```python
from build123d import *

# Parameters (mm, degrees)
EXTRUDE_1_DEPTH     = 3
SKETCH_2_R          = 2.5
CUT_EXTRUDE_1_DEPTH = 3


with BuildPart() as part:
    # 草图1 → 凸台-拉伸1 (new body)
    with BuildSketch(Plane(origin=(0, 0, 0), x_dir=(1, 0, 0), z_dir=(0, 1, 0))):
        with BuildLine():
            ThreePointArc((6.796232726, -80.103971167), (3.309364716, -83.445468492), (6.479618851, -87.088728243))
            ThreePointArc((6.479618851, -87.088728243), (23.201931583, -85.196198653), (37.766812343, -76.765204654))
            ThreePointArc((37.766812343, -76.765204654), (38.146329718, -71.950662158), (33.355557274, -71.3404554))
            ThreePointArc((33.355557274, -71.3404554), (20.773998873, -77.837935766), (6.796232726, -80.103971167))
        make_face()
    extrude(amount=EXTRUDE_1_DEPTH)

    # 草图2 → 切除-拉伸1 (cut)
    with BuildSketch(Plane(origin=(0, 0, 0), x_dir=(1, 0, 0), z_dir=(0, 1, 0))):
        with Locations(Location((6.805774449, -83.603958161, 0), (0, 0, 270))):
            Circle(SKETCH_2_R)
        with Locations(Location((35.430824241, -74.158835612, 0), (0, 0, 270))):
            Circle(SKETCH_2_R)
    extrude(amount=CUT_EXTRUDE_1_DEPTH, mode=Mode.SUBTRACT)


solid = part.part
```
The model under review builds one solid part; all positions refer to its coordinate system, in mm. Round coordinates to 2 decimals unless told otherwise and drop trailing zeros. Loops run counter-clockwise (first coordinate to the right, second up) from the corner with the lowest first, then second, coordinate; pieces in that order, holes last. Notation, with made-up numbers: M 50,-18.75 L 104,-18.75 A16 cw 104,1.25 Z; hole C 23,-25 d5. An arc over 180 degrees is marked long. Write item = value, one per line.
Item 1: Take a section at C-C on y = 2.65. Write out the cut boundary in (x, z).
Return value:
outline = M 6.48,87.09 A3.5 ccw 6.8,80.1 A45 cw 33.36,71.34 A3.5 ccw 37.77,76.77 A41.13 ccw Z; hole C 6.81,83.6 d5; hole C 35.43,74.16 d5
Item 2: Take a section at B-B on x = 5. Write out the cut boundary in (y, z).
Return value:
outline = M 0,80.61 L 3,80.61 L 3,81.88 L 0,81.88 Z; M 0,85.33 L 3,85.33 L 3,86.6 L 0,86.6 Z
Item 3: For line 1 (X direction, y = 1.2, z = 83.5); line 2 (X direction, y = 0.95, z = 76.25); line 3 (Z direction, x = 36.5, y = 1.55), list the stretches that pass through material, from the lowest coordinate up. Write a range as [from, to].
Return value:
line_1 = [3.31, 4.31], [9.3, 27.51]
line_2 = [24.89, 34.06], [36.8, 38.24]
line_3 = [70.83, 71.9], [76.42, 77.86]
Item 4: Take a section at D-D on x = 20. Write out the cut boundary in (y, z).
Return value:
outline = M 0,78.09 L 3,78.09 L 3,86.11 L 0,86.11 Z
Item 5: The part is to be moulded in two halves that separate along Z. For faces 1 (the flat face through (21, 3, 81)), 2 (the cylindrical face through (7.557, 1.479, 85.989)), 3 (the cylindrical face through (22.98, 1.48, 85.27)), say which applies: released by +Z, released by -Z, zero draft, split by the parting line, or undercut.
Return value:
face_1 = zero draft
face_2 = undercut
face_3 = released by +Z
Item 6: Insertion check: P1, Ø4, axis at x = 35.43, z = 74.16, coming from the +Y side; P2, Ø1.5, axis at x = 27, y = 2.5, coming from the +Z side. Each pin has a flat end and moves straight along its axis. Give the tip position at first contact, or say it passes through.
Return value:
P1 = through
P2 = 84.05
Item 7: Take a section at A-A on z = 75. Write out the cut boundary in (x, y), then the cut area to 3 significant figures.
Return value:
outline = M 27.49,0 L 33.08,0 L 33.08,3 L 27.49,3 Z; M 37.79,0 L 38.83,0 L 38.83,3 L 37.79,3 Z
area = 19.9 mm2
